The listing builds one solid part. Answer for the finished solid, in the listing's coordinates (mm). Face numbers are marked on the shaded views. A direction names the side the tool comes from. Coordinates: 2 decimals unless noted, no trailing zeros. Write each loop counter-clockwise with the first axis right and the second up, starting at its lowest first coordinate (ties: lowest second). Pieces come first, ordered by that corner, then holes.
Autodesk Inventor part; units mm, degrees
ref_plane "YZ Plane" through (0, 0, 0) normal (1, 0, 0) x (0, 1, 0)
ref_plane "XZ Plane" through (0, 0, 0) normal (0, 1, 0) x (-1, 0, 0)
ref_plane "XY Plane" through (0, 0, 0) normal (0, 0, 1) x (1, 0, 0)
sketch "Esboço8" plane through (0, 0, 0) normal (0, 1, 0) x (-1, 0, 0)
  line L0 (0, 0) -> (-80, 0)
  line L1 (-80, 0) -> (-80, -70)
  line L2 (-80, -70) -> (0, -70)
  line L3 (0, -70) -> (0, 0)
  line L4 (0, 0) -> (-18, 0)
  line L5 (-80, -70) -> (-62, -70)
  line L6 (-18, 0) -> (-62, 0)
  line L7 (-62, 0) -> (-62, -70)
  line L8 (-62, -70) -> (-18, -70)
  line L9 (-18, -70) -> (-18, 0)
  dimension "d19" = 80
  dimension "d20" = 70
  dimension "d21" = 18
  dimension "d22" = 18
extrude "Extrusão6" add sketch "Esboço8" along normal blind 5 contours L3 L2 L9 L0 | L7 L2 L1 L0
sketch "Esboço9" plane through (0, 0, 0) normal (0, -1, 0) x (1, 0, 0)
  line L0 (0, 0) -> (18, 0)
  line L1 (62, -70) -> (62, 0)
  line L2 (18, 0) -> (62, 0)
  line L3 (62, 0) -> (62, -70)
  line L4 (62, -70) -> (18, -70)
  line L5 (18, -70) -> (18, 0)
extrude "Extrusão7" add sketch "Esboço9" against normal blind 46
sketch "Esboço10" plane through (0, 0, 0) normal (0, -1, 0) x (1, 0, 0)
  line L0 (18, 0) -> (62, 0)
  line L1 (62, -70) -> (62, 0)
  line L2 (18, 0) -> (62, 0)
  line L3 (62, 0) -> (62, -70)
  line L4 (62, -70) -> (18, -70)
  line L5 (18, -70) -> (18, 0)
  line L6 (0, 0) -> (18, 0)
  line L7 (18, 0) -> (23, 0)
  line L8 (23, 0) -> (23, -5)
  line L9 (23, -5) -> (18, -5)
  line L10 (18, -5) -> (18, 0)
  line L11 (62, -70) -> (57, -70)
  line L12 (57, -70) -> (57, -65)
  line L13 (57, -65) -> (62, -65)
  line L14 (62, -65) -> (62, -70)
  line L15 (23, -5) -> (57, -5)
  line L16 (57, -5) -> (57, -65)
  line L17 (57, -65) -> (23, -65)
  line L18 (23, -65) -> (23, -5)
  dimension "d27" = 5
  dimension "d28" = 5
  dimension "d29" = 5
  dimension "d30" = 5
extrude "Extrusão8" cut sketch "Esboço10" against normal blind 40 contours L15 L16 L17 L18
fillet "Arredondamento1" radius 5 16 edges at (62, 46, -35) (40, 46, 0) (18, 25.5, 0) (62, 25.5, 0) (62, 5, -35) (62, 25.5, -70) (80, 5, -35) (40, 46, -70) (18, 46, -35) (18, 25.5, -70) (18, 5, -35) (9, 5, -70) (9, 5, 0) (0, 5, -35) (71, 5, -70) (71, 5, 0)
sketch "Esboço11" plane through (0, 46, 0) normal (0, 1, 0) x (1, 0, 0)
  line L0 (23, 65) -> (23, 5)
  line L1 (57, 5) -> (57, 65)
  line L2 (23, 5) -> (57, 5)
  line L3 (57, 5) -> (57, 65)
  line L4 (57, 65) -> (23, 65)
  line L5 (23, 65) -> (23, 5)
  line L6 (40, 65) -> (40, 51.3)
  circle A0 centre (40, 51.3) radius 13
  point P0 (0, 0)
  dimension "d34" = 13.7
  dimension "d35" = 26
extrude "Extrusão9" cut sketch "Esboço11" against normal blind 10 contours A0
properties part number "case_motor_inferior"
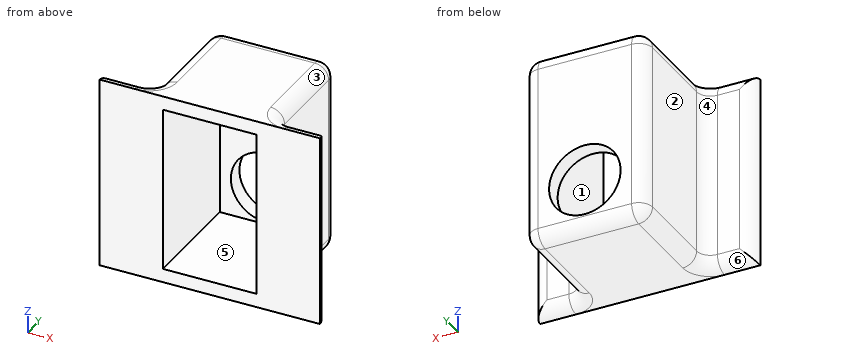
Q1. Which of the six approach directions +Z, -Z, +X, -X, +Y, -Y give full straight-line access (tool end or side, diameter ignored) to the marked faces 1, 2 and 3?
Answers below:
face 1: -Y
face 2: +Z, -Z, -X, +Y
face 3: +Z, +X, +Y
Q2. Given pin 1 (23.5 mm diameter, centred on x = 40, z = -51.3, fed in from -Y); pin 2 (12 mm diameter, centred on y = 28.5, z = -47, fed in from +X); pin 3 (9 mm diameter, centred on x = 8, z = -35, fed in from +Y); pin 4 (4 mm diameter, centred on x = 68, y = 5.5, fed in from +Z), each flat-ended and moving along its own axis, determine where each tip first touches the part or whether it passes through.
Answers below:
pin 1: passes through
pin 2: stops at x = 62
pin 3: stops at y = 5
pin 4: stops at z = -1.43
Q3. Determine the mould class of the marked faces 4, 5 and 6 for opening direction Z: released by +Z, released by -Z, zero draft, split by the parting line, or undercut.
Answers below:
face 4: zero draft
face 5: undercut
face 6: released by -Z
Q4. The part is cut by section C-C, the plane y = 20. Write down the section's boundary in (x, z).
Answers below:
outline: (18, -65) arc R5 ccw to (23, -70) - (57, -70) arc R5 ccw to (62, -65) - (62, -5) arc R5 ccw to (57, 0) - (23, 0) arc R5 ccw to (18, -5) - close; hole (23, -65) - (57, -65) - (57, -5) - (23, -5) - close
Q5. Find the intervals of material crossed by probe 1 along Z at (x, y) = (48, 38.5); probe 2 along X at (y, z) = (22.5, -55); probe 3 along Y at (x, z) = (33, -63), in increasing order.
Answers below:
probe 1: z = -70 to -65, -5 to 0
probe 2: x = 18 to 23, 57 to 62
probe 3: y = 40 to 46
Q6. The part is cut by section A-A, the plane x = 40. Write down the section's boundary in (y, z), then the cut area to 3 significant figures.
Answers below:
outline: (0, -70) - (41, -70) arc R5 ccw to (46, -65) - (46, -64.3) - (40, -64.3) - (40, -65) - (0, -65) - close; (0, -5) - (40, -5) - (40, -38.3) - (46, -38.3) - (46, -5) arc R5 ccw to (41, 0) - (0, 0) - close
area: 653 mm2
